Geometry check sheet. Reference: the model listing, model coordinates, mm. Face numbers are marked on the shaded views. A direction names the side the tool comes from. Round coordinates to 2 decimals unless told otherwise and drop trailing zeros. Write each loop counter-clockwise with the first axis right and the second up, starting at its lowest first coordinate (ties: lowest second). Pieces come first, ordered by that corner, then holes. Notation, with made-up numbers: M 21,82 L 33,82 A17 cw 33,98 Z; hole C 80.5,62.5 d7. An arc over 180 degrees is marked long. One line per item, written item: value. Start each with the question number.
1. Section check B-B (z = 5). Record the boundary of the cut face in (x, y).
2. Section check A-A (x = 0). Record the boundary of the cut face in (y, z), and give its area (3 significant figures).
3. Scan lines: probe 1 along X at (y, z) = (-32.5, -12); probe 2 along X at (y, z) = (1, 1); probe 3 along X at (y, z) = (0.5, -4). Record each from-to range of solid material in increasing order. Write a range as [from, to].
4. Access from +Z, -Z, +X, -X, +Y, -Y to the whole of each face (thin tool, end or side, straight path). Record for the marked faces 1 and 2.
5. Depth check by flat-ended pin: P1, Ø4, axis at x = 44.5, z = 4.5, coming from the -Y side; P2, Ø6, axis at y = -17, z = -7, coming from the +X side; P3, Ø1.5, axis at y = 2.5, z = -16.5, coming from the +X side; P4, Ø8, axis at x = -7, y = 5.5, coming from the -Z side. Enter the tip coordinate at first touch or a pass-through.
6. Release check for a two-part mould opening along X. For the marked faces 3, 4 and 5 record: pulls with the +X half, pulls with the -X half, needs draft (parallel to the pull), parting line crosses it, or undercut.
7. Section check D-D (z = -3). Record the boundary of the cut face in (x, y), and give its area (3 significant figures).
8. Section check C-C (y = -11). Record the boundary of the cut face in (x, z).
from build123d import *

# Parameters (mm, degrees)
IZIM1_R                     = 62.2
Y_KSEKLIK_EKSTR_ZYON3_DEPTH = 10
Y_KSEKLIK_EKSTR_ZYON4_START = 20
IZIM2_R                     = 62.2
Y_KSEKLIK_EKSTR_ZYON4_DEPTH = 20
IZIM12_R                    = 15
KES_EKSTR_ZYON1_DEPTH       = 93.939119858
DAIRESEL_KAPLAMA1_COUNT     = 10


with BuildPart() as part:
    # Çizim1 → Yükseklik-Ekstrüzyon3 (new body)
    with BuildSketch(Plane.XY):
        Circle(IZIM1_R)
        with BuildLine():
            Line((31.5, 47), (-31.5, 47))
            ThreePointArc((-31.5, 47), (-33.08113883, 46.74341649), (-34.5, 46))
            ThreePointArc((-34.5, 46), (-57.5, 0), (-34.5, -46))
            ThreePointArc((-34.5, -46), (-33.08113883, -46.74341649), (-31.5, -47))
            Line((-31.5, -47), (31.5, -47))
            ThreePointArc((31.5, -47), (33.08113883, -46.74341649), (34.5, -46))
            ThreePointArc((34.5, -46), (57.5, 0), (34.5, 46))
            ThreePointArc((34.5, 46), (33.08113883, 46.74341649), (31.5, 47))
        make_face(mode=Mode.SUBTRACT)
    extrude(amount=Y_KSEKLIK_EKSTR_ZYON3_DEPTH)

    # Çizim2 → Yükseklik-Ekstrüzyon4 (add)
    with BuildSketch(Plane(origin=(0, 0, 0), x_dir=(-1, 0, 0), z_dir=(0, 0, -1)).offset(Y_KSEKLIK_EKSTR_ZYON4_START)):
        Circle(IZIM2_R)
    extrude(amount=-Y_KSEKLIK_EKSTR_ZYON4_DEPTH)

    # Çizim12 → Kes-Ekstrüzyon1 (cut, through all)
    with BuildSketch(Plane.XY.offset(10)):
        Circle(IZIM12_R)
        Polygon((-50.603744818, 50), (50.603744818, 50), (-3.038589064, 77.096458803), align=None)
        Polygon((36.997837775, -50), (-36.997837775, -50), (-1.176281375, -79.482501569), align=None)
    extrude(amount=-KES_EKSTR_ZYON1_DEPTH, mode=Mode.SUBTRACT)

    # Çizim15 → M5x0.8 Helisarmal İçin Dişli Delik1 (revolve, cut)
    with BuildSketch(Plane(origin=(62.2, 0, -10), x_dir=(0, 0, -1), z_dir=(0, 1, 0))):
        Polygon((0, 0), (0, 15.162237609), (2.6, 13.6), (2.6, 0), align=None)
    m5x0_8_helisarmal_in_di_li_delik1 = revolve(axis=Axis((68.55, 0, -10), (-1, 0, 0)), mode=Mode.SUBTRACT)

    # Dairesel Kaplama1: M5x0.8 Helisarmal İçin Dişli Delik1 ×10 about axis, 4 skipped
    dairesel_kaplama1_axis = Axis((0, 0, 10), (0, 0, 1))
    add([m5x0_8_helisarmal_in_di_li_delik1.rotate(dairesel_kaplama1_axis, i * 360 / DAIRESEL_KAPLAMA1_COUNT) for i in range(1, DAIRESEL_KAPLAMA1_COUNT) if i not in (2, 3, 7, 8)], mode=Mode.SUBTRACT)


solid = part.part
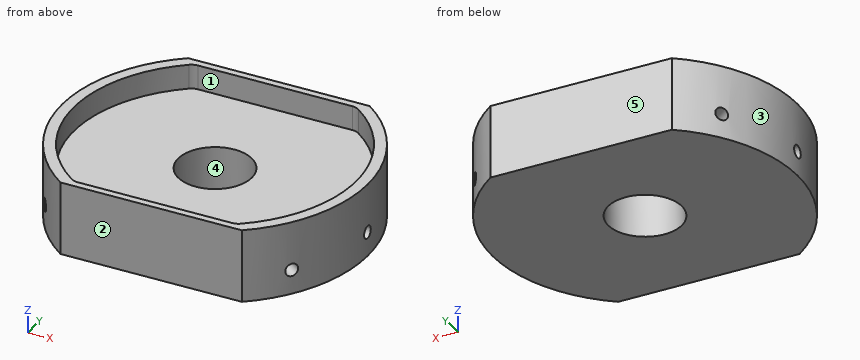
Result sheet:
1. outline: M -37,-50 L 37,-50 A62.2 ccw 37,50 L -37,50 A62.2 ccw Z; hole M -34.5,-46 A5 ccw -31.5,-47 L 31.5,-47 A5 ccw 34.5,-46 A57.5 ccw 34.5,46 A5 ccw 31.5,47 L -31.5,47 A5 ccw -34.5,46 A57.5 ccw Z
2. outline: M -50,-20 L -15,-20 L -15,0 L -47,0 L -47,10 L -50,10 Z; M 15,-20 L 50,-20 L 50,10 L 47,10 L 47,0 L 15,0 Z
2. area: 1,460 mm2
3. probe 1: x = [-53.03, -47.56], [-41.91, 41.91], [47.56, 53.03]
3. probe 2: x = [-62.19, -57.49], [57.49, 62.19]
3. probe 3: x = [-62.2, -14.99], [14.99, 62.2]
4. face 1: +Z
4. face 2: +Z, -Z, +X, -X, -Y
5. P1: stops at y = -45.42
5. P2: stops at x = 60.6
5. P3: stops at x = 62.18
5. P4: passes through
6. face 3: pulls with the -X half
6. face 4: undercut
6. face 5: needs draft
7. outline: M -37,-50 L 37,-50 A62.2 ccw 37,50 L -37,50 A62.2 ccw Z; hole C 0,0 d30
7. area: 10,200 mm2
8. outline: M -61.22,-20 L -10.2,-20 L -10.2,0 L -56.44,0 L -56.44,10 L -61.22,10 Z; M 10.2,-20 L 61.22,-20 L 61.22,10 L 56.44,10 L 56.44,0 L 10.2,0 Z
